from build123d import *

# Parameters (mm, degrees)
SKETCH1_W                                    = 50
SKETCH1_H                                    = 110
BOSS_EXTRUDE1_DEPTH                          = 5
CBORE_FOR_M3_HEXAGON_SOCKET_HEAD_CAP_2_COUNT = 2
CBORE_FOR_M3_HEXAGON_SOCKET_HEAD_CAP_2_PITCH = 43.5
CBORE_FOR_M3_HEXAGON_SOCKET_HEAD_CAP_3_COUNT = 2
CBORE_FOR_M3_HEXAGON_SOCKET_HEAD_CAP_3_PITCH = 100
CBORE_FOR_M3_HEXAGON_SOCKET_HEAD_CAP_4_COUNT = 2
CBORE_FOR_M3_HEXAGON_SOCKET_HEAD_CAP_4_PITCH = 109.051593294
SKETCH5_W                                    = 35
SKETCH5_H                                    = 85
CUT_EXTRUDE1_DEPTH                           = 61.621778265
FILLET1_R                                    = 4


with BuildPart() as part:
    # Sketch1 → Boss-Extrude1 (new body)
    with BuildSketch(Plane(origin=(0, 0, 0), x_dir=(1, 0, 0), z_dir=(0, 1, 0))):
        Rectangle(SKETCH1_W, SKETCH1_H)
    extrude(amount=BOSS_EXTRUDE1_DEPTH)

    # Sketch4 → CBORE for M3 Hexagon socket head cap screws1 (revolve, cut)
    with BuildSketch(Plane(origin=(-21.75, 5, -50), x_dir=(0, 0, 1), z_dir=(1, 0, 0))):
        Polygon((0, 0), (0, 10.96137699), (1.6, 10), (1.6, 3.4), (3, 3.4), (3, 0.025), (3.025, 0), align=None)
    cbore_for_m3_hexagon_socket_head_cap_scr = revolve(axis=Axis((-21.75, 11.35, -50), (0, -1, 0)), mode=Mode.SUBTRACT)

    # CBORE for M3 Hexagon socket head cap 2: CBORE for M3 Hexagon socket head cap screws1 ×2
    with Locations(*[(i * CBORE_FOR_M3_HEXAGON_SOCKET_HEAD_CAP_2_PITCH, 0, 0) for i in range(1, CBORE_FOR_M3_HEXAGON_SOCKET_HEAD_CAP_2_COUNT)]):
        add(cbore_for_m3_hexagon_socket_head_cap_scr, mode=Mode.SUBTRACT)

    # CBORE for M3 Hexagon socket head cap 3: CBORE for M3 Hexagon socket head cap screws1 ×2
    with Locations(*[(0, 0, i * CBORE_FOR_M3_HEXAGON_SOCKET_HEAD_CAP_3_PITCH) for i in range(1, CBORE_FOR_M3_HEXAGON_SOCKET_HEAD_CAP_3_COUNT)]):
        add(cbore_for_m3_hexagon_socket_head_cap_scr, mode=Mode.SUBTRACT)

    # CBORE for M3 Hexagon socket head cap 4: CBORE for M3 Hexagon socket head cap screws1 ×2
    with Locations(*[Vector(0.3988937592379055, 0, 0.9169971476733457) * (i * CBORE_FOR_M3_HEXAGON_SOCKET_HEAD_CAP_4_PITCH) for i in range(1, CBORE_FOR_M3_HEXAGON_SOCKET_HEAD_CAP_4_COUNT)]):
        add(cbore_for_m3_hexagon_socket_head_cap_scr, mode=Mode.SUBTRACT)

    # Sketch5 → Cut-Extrude1 (cut, through all)
    with BuildSketch(Plane(origin=(0, 5, 0), x_dir=(1, 0, 0), z_dir=(0, 1, 0))):
        Rectangle(SKETCH5_W, SKETCH5_H)
    extrude(amount=-CUT_EXTRUDE1_DEPTH, mode=Mode.SUBTRACT)

    # Fillet1
    fillet1_edges = [part.edges().sort_by_distance(p)[0] for p in [
        (-17.5, 2.5, 42.5),
        (-17.5, 2.5, -42.5),
        (17.5, 2.5, -42.5),
        (17.5, 2.5, 42.5),
    ]]
    fillet(fillet1_edges, radius=FILLET1_R)


solid = part.part
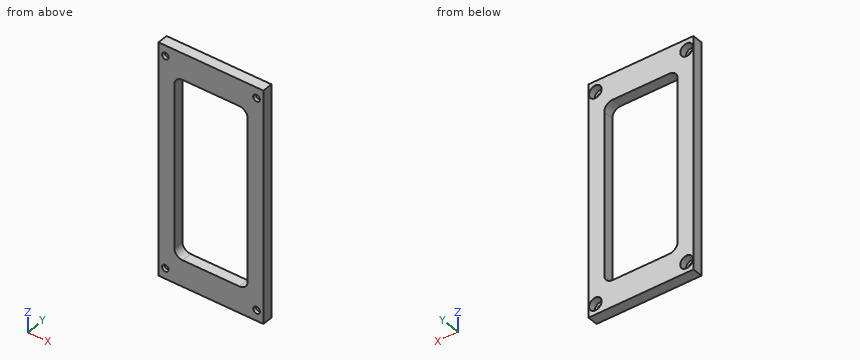
For this review, take the finished solid that the model builds, in its own axes (mm). Round coordinates to 2 decimals unless told otherwise and drop trailing zeros. Write each loop counter-clockwise with the first axis right and the second up, starting at its lowest first coordinate (ties: lowest second). Pieces come first, ordered by that corner, then holes. Notation, with made-up numbers: (-1.5, 25) -> (5.5, 25) arc R17 cw to (5.5, 50) -> close; hole circle Ø4 at (87, 43.25). An arc over 180 degrees is marked (long way). Use CSV: the item, a comma, the result in double quotes.
(1) To check wall thickness, follow L1, parallel to Z at x = 21.75, y = 3.4; L2, parallel to Z at x = 21.75, y = 0.55; L3, parallel to X at y = 2.95, z = -50. State the ranges of each line that lie inside material, in increasing order. Write a range as [from, to].
Computed values:
L1,"[-55, -53], [-47, 47], [53, 55]"
L2,"[-55, -51.6], [-48.4, 48.4], [51.6, 55]"
L3,"[-25, -24.75], [-18.75, 18.75], [24.75, 25]"
(2) Consider section B-B, the plane z = -6. Give the boundary of the cut face in (x, y), plus the area to 3 significant figures.
Computed values:
outline,"(-25, 0) -> (-17.5, 0) -> (-17.5, 5) -> (-25, 5) -> close; (17.5, 0) -> (25, 0) -> (25, 5) -> (17.5, 5) -> close"
area,"75.0 mm²"
(3) Consider section A-A, the plane z = 50. Give the boundary of the cut face in (x, y) (3 decimals).
Computed values:
outline,"(-25, 0) -> (-23.35, 0) -> (-23.35, 1.6) -> (-24.75, 1.6) -> (-24.75, 4.975) -> (-24.775, 5) -> (-25, 5) -> close; (-20.15, 0) -> (20.15, 0) -> (20.15, 1.6) -> (18.75, 1.6) -> (18.75, 4.975) -> (18.725, 5) -> (-18.725, 5) -> (-18.75, 4.975) -> (-18.75, 1.6) -> (-20.15, 1.6) -> close; (23.35, 0) -> (25, 0) -> (25, 5) -> (24.775, 5) -> (24.75, 4.975) -> (24.75, 1.6) -> (23.35, 1.6) -> close"
(4) Consider section C-C, the plane x = 9.5. Give the boundary of the cut face in (y, z), plus the area to 3 significant figures.
Computed values:
outline,"(0, -55) -> (5, -55) -> (5, -42.5) -> (0, -42.5) -> close; (0, 42.5) -> (5, 42.5) -> (5, 55) -> (0, 55) -> close"
area,"125 mm²"
(5) Clearance check with flat-ended pins moving along their axes: P1, Ø3, axis at x = -21.5, z = -50.5, coming from the +Y side; P2, Ø3, axis at x = 21.75, z = -50, coming from the +Y side. State where each tip first meets the part, or that it passes through.
Computed values:
P1,"y = 1.6"
P2,"through"
(6) Consider section D-D, the plane y = 4.15. Give the boundary of the cut face in (x, z), plus the area to 3 significant figures.
Computed values:
outline,"(-25, -55) -> (25, -55) -> (25, 55) -> (-25, 55) -> close; hole circle Ø6 at (-21.75, -50); hole circle Ø6 at (-21.75, 50); hole (-17.5, -38.5) arc R4 ccw to (-13.5, -42.5) -> (13.5, -42.5) arc R4 ccw to (17.5, -38.5) -> (17.5, 38.5) arc R4 ccw to (13.5, 42.5) -> (-13.5, 42.5) arc R4 ccw to (-17.5, 38.5) -> close; hole circle Ø6 at (21.75, -50); hole circle Ø6 at (21.75, 50)"
area,"2,430 mm²"
